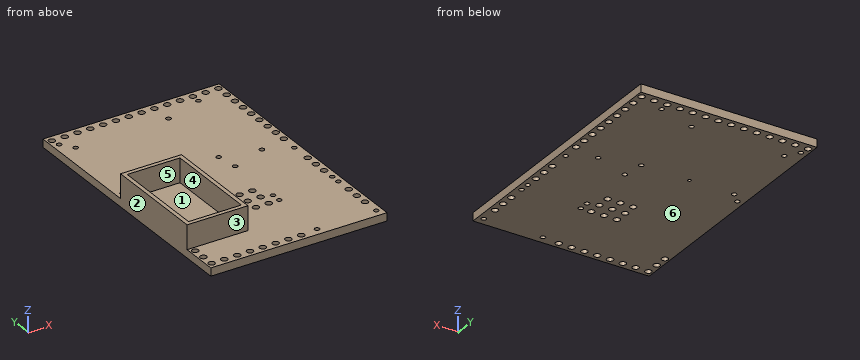
Autodesk Fusion 360 part; units mm, degrees
sketch "Skizze1" plane through (0, 0, 0) normal (0, 0, 1) x (1, 0, 0)
  line L0 (-55, 110) -> (55, 110)
  line L1 (55, 110) -> (55, -50)
  line L2 (55, -50) -> (-55, -50)
  line L3 (-55, -50) -> (-55, 110)
  circle A0 centre (0, 0) radius 2
  line L4 (0, 0) -> (-8, 0)
  line L5 (-8, 0) -> (-8, 8)
  line L6 (-8, 8) -> (0, 8)
  line L7 (0, 8) -> (0, 0)
  line L8 (-8, 8) -> (8, 8)
  line L9 (8, 8) -> (8, -8)
  line L10 (8, -8) -> (-8, -8)
  line L11 (-8, -8) -> (-8, 8)
  line L12 (0, 8) -> (8, 8)
  line L13 (8, 8) -> (8, -8)
  line L14 (8, -8) -> (0, -8)
  line L15 (0, -8) -> (0, 8)
  line L16 (-8, 0) -> (8, 0)
  line L17 (8, 0) -> (8, -8)
  line L18 (8, -8) -> (-8, -8)
  line L19 (-8, -8) -> (-8, 0)
  circle A1 centre (0, 8) radius 2
  circle A2 centre (-8, 8) radius 2
  circle A3 centre (-8, 0) radius 2
  circle A4 centre (-8, -8) radius 2
  circle A5 centre (0, -8) radius 2
  circle A6 centre (8, -8) radius 2
  circle A7 centre (8, 0) radius 2
  circle A8 centre (8, 8) radius 2
  circle A9 centre (-45.5, 97) radius 1.5
  circle A10 centre (12.5, 48) radius 1.5
  line L20 (-45.5, 97) -> (12.5, 97)
  line L21 (12.5, 97) -> (12.5, 48)
  line L22 (12.5, 48) -> (-45.5, 48)
  line L23 (-45.5, 48) -> (-45.5, 97)
  circle A11 centre (-45.5, 48) radius 1.5
  circle A12 centre (12.5, 97) radius 1.5
  line L24 (-50, 101.5) -> (35, 101.5)
  line L25 (35, 101.5) -> (35, 45.5)
  line L26 (35, 45.5) -> (-50, 45.5)
  line L27 (-50, 45.5) -> (-50, 101.5)
  line L28 (-45.5, 48) -> (12.5, 48)
  line L29 (12.5, 48) -> (12.5, 72.5)
  line L30 (-50, 45.5) -> (35, 45.5)
  line L31 (35, 45.5) -> (35, 73.5)
  line L32 (-51, 104.5) -> (36, 104.5)
  line L33 (36, 104.5) -> (36, 42.5)
  line L34 (36, 42.5) -> (-51, 42.5)
  line L35 (-51, 42.5) -> (-51, 104.5)
  circle A13 centre (-51, 42.5) radius 1.5
  circle A14 centre (-51, 104.5) radius 1.5
  circle A15 centre (36, 104.5) radius 1.5
  circle A16 centre (36, 42.5) radius 1.5
  line L36 (-7.5, 104.5) -> (-7.5, 42.5)
  line L37 (36, 73.5) -> (-51, 73.5)
  line L38 (-7.5, 101.5) -> (-7.5, 45.5)
  line L39 (35, 73.5) -> (-50, 73.5)
  line L40 (-52.5, 35.7098) -> (-19.5, 35.7098)
  line L41 (-19.5, 35.7098) -> (-19.5, -24.2902)
  line L42 (-19.5, -24.2902) -> (-52.5, -24.2902)
  line L43 (-52.5, -24.2902) -> (-52.5, 35.7098)
  line L44 (-36, 35.7098) -> (-36, -24.2902)
  line L45 (-19.5, 5.7098) -> (-52.5, 5.7098)
  line L46 (-55, 38.2098) -> (-17, 38.2098)
  line L47 (-17, 38.2098) -> (-17, -26.7902)
  line L48 (-17, -26.7902) -> (-55, -26.7902)
  line L49 (-55, -26.7902) -> (-55, 38.2098)
  line L50 (-36, 38.2098) -> (-36, -26.7902)
  line L51 (-17, 5.7098) -> (-55, 5.7098)
  line L52 (11.5, -5) -> (54.5, -5)
  line L53 (54.5, -5) -> (54.5, -48)
  line L54 (54.5, -48) -> (11.5, -48)
  line L55 (11.5, -48) -> (11.5, -5)
  line L56 (14.5, -8) -> (51.5, -8)
  line L57 (51.5, -8) -> (51.5, -45)
  line L58 (51.5, -45) -> (14.5, -45)
  line L59 (14.5, -45) -> (14.5, -8)
  circle A17 centre (14.5, -8) radius 1.5
  circle A18 centre (51.5, -8) radius 1.5
  circle A19 centre (51.5, -45) radius 1.5
  circle A20 centre (14.5, -45) radius 1.5
  line L60 (14.5, -26.5) -> (51.5, -26.5)
  line L61 (33, -8) -> (33, -45)
  line L62 (33, -5) -> (33, -48)
  line L63 (54.5, -26.5) -> (11.5, -26.5)
  line L64 (11.5, -5) -> (11.5, 38)
  circle A21 centre (14.5, -2) radius 1.5
  circle A22 centre (51.5, 35) radius 1.5
  circle A23 centre (14.5, 35) radius 1.5
  line L65 (11.5, 38) -> (54.5, 38)
  line L66 (33, 38) -> (33, -5)
  line L67 (54.5, 16.5) -> (11.5, 16.5)
  line L68 (33, 35) -> (33, -2)
  line L69 (14.5, 16.5) -> (51.5, 16.5)
  line L70 (14.5, 35) -> (51.5, 35)
  line L71 (54.5, -5) -> (11.5, -5)
  line L72 (51.5, 35) -> (51.5, -2)
  line L73 (54.5, 38) -> (54.5, -5)
  line L74 (51.5, -2) -> (14.5, -2)
  circle A24 centre (51.5, -2) radius 1.5
  line L75 (14.5, -2) -> (14.5, 35)
  line L76 (33, 16.5) -> (33, -26.5)
  line L77 (-55, 110) -> (55, 110)
  line L78 (55, 110) -> (55, 104.5)
  line L79 (55, 104.5) -> (-55, 104.5)
  line L80 (-55, 104.5) -> (-55, 110)
  line L81 (-55, 104.5) -> (-7.5, 104.5)
  line L82 (-7.5, 104.5) -> (-7.5, 73.5)
  line L83 (-7.5, 73.5) -> (-55, 73.5)
  line L84 (-55, 73.5) -> (-55, 104.5)
  line L85 (-55, 42.7098) -> (-36, 42.7098)
  line L86 (-36, 42.7098) -> (-36, 5.7098)
  line L87 (-36, 5.7098) -> (-55, 5.7098)
  line L88 (-55, 5.7098) -> (-55, 42.7098)
  line L89 (55, 42.5) -> (33, 42.5)
  line L90 (33, 42.5) -> (33, 16.5)
  line L91 (33, 16.5) -> (55, 16.5)
  line L92 (55, 16.5) -> (55, 42.5)
  line L93 (-55, 110) -> (55, 110)
  line L94 (55, 110) -> (55, 114)
  line L95 (55, 114) -> (-55, 114)
  line L96 (-55, 114) -> (-55, 110)
  circle A25 centre (-28, 110) radius 2
  circle A26 centre (-20, 110) radius 2
  circle A27 centre (-12, 110) radius 2
  circle A28 centre (-36, 110) radius 2
  circle A29 centre (-44, 110) radius 2
  circle A30 centre (-52, 110) radius 2
  circle A31 centre (-4, 110) radius 2
  circle A32 centre (4, 110) radius 2
  circle A33 centre (12, 110) radius 2
  circle A34 centre (20, 110) radius 2
  circle A35 centre (28, 110) radius 2
  circle A36 centre (36, 110) radius 2
  circle A37 centre (44, 110) radius 2
  circle A38 centre (52, 110) radius 2
  line L97 (52, 110) -> (52, 42.5)
  circle A39 centre (52, 102) radius 2
  circle A40 centre (52, 94) radius 2
  circle A41 centre (52, 86) radius 2
  circle A42 centre (52, 70) radius 2
  circle A43 centre (52, 78) radius 2
  circle A44 centre (52, 62) radius 2
  circle A45 centre (52, 54) radius 2
  circle A46 centre (52, 46) radius 2
  line L98 (-55, -50) -> (11.5, -50)
  line L99 (11.5, -50) -> (11.5, -46)
  line L100 (11.5, -46) -> (-55, -46)
  line L101 (-55, -46) -> (-55, -50)
  circle A47 centre (-52, -46) radius 2
  circle A48 centre (-44, -46) radius 2
  circle A49 centre (-36, -46) radius 2
  circle A50 centre (-28, -46) radius 2
  circle A51 centre (-20, -46) radius 2
  circle A52 centre (-12, -46) radius 2
  circle A53 centre (-4, -46) radius 2
  circle A54 centre (4, -46) radius 2
  circle A55 centre (-17.5, 48) radius 1
  line L102 (-52, -46) -> (-52, -24.2902)
  circle A56 centre (-52, -38) radius 2
  circle A57 centre (-52, -30) radius 2
  circle A58 centre (51.5, 22) radius 2
  circle A59 centre (51.5, 14) radius 2
  circle A60 centre (51.5, 6) radius 2
  circle A61 centre (51.5, -18) radius 2
  circle A62 centre (51.5, -26) radius 2
  circle A63 centre (51.5, -34) radius 2
  point P0 (-7.5, 73.5)
  point P1 (-7.5, 73.5)
  point P2 (-36, 5.7098)
  point P3 (-36, 5.7098)
  point P4 (33, -26.5)
  point P5 (33, -26.5)
  point P6 (33, 16.5)
  point P7 (33, 16.5)
  point P8 (-52, 110)
  point P9 (-44, 110)
  point P10 (-36, 110)
  dimension "d1" = 110
  dimension "d2" = 160
  dimension "d3" = 55
  dimension "d4" = 50
  dimension "d5" = 4
  dimension "d6" = 8
  dimension "d7" = 8
  dimension "d8" = 16
  dimension "d9" = 16
  dimension "d10" = 4
  dimension "d11" = 4
  dimension "d12" = 4
  dimension "d13" = 4
  dimension "d14" = 4
  dimension "d15" = 4
  dimension "d16" = 4
  dimension "d17" = 4
  dimension "d20" = 3
  dimension "d23" = 3
  dimension "d28" = 3
  dimension "d29" = 3
  dimension "d30" = 58
  dimension "d31" = 49
  dimension "d32" = 85
  dimension "d33" = 56
  dimension "d35" = 4.5
  dimension "d36" = 4.5
  dimension "d37" = 87
  dimension "d38" = 62
  dimension "d39" = 3
  dimension "d40" = 3
  dimension "d41" = 3
  dimension "d42" = 3
  dimension "d45" = 33
  dimension "d46" = 60
  dimension "d47" = 38
  dimension "d48" = 65
  dimension "d51" = 43
  dimension "d52" = 43
  dimension "d53" = 37
  dimension "d54" = 37
  dimension "d55" = 3
  dimension "d56" = 3
  dimension "d57" = 3
  dimension "d58" = 3
  dimension "d59" = 43
  dimension "d60" = 43
  dimension "d61" = 37
  dimension "d62" = 37
  dimension "d63" = 3
  dimension "d64" = 3
  dimension "d65" = 3
  dimension "d66" = 3
  dimension "d67" = 43
  dimension "d68" = 5.5
  dimension "d69" = 47.5
  dimension "d70" = 31
  dimension "d71" = 19
  dimension "d72" = 37
  dimension "d73" = 22
  dimension "d74" = 26
  dimension "d75" = 4
  dimension "d76" = 3
  dimension "d77" = 8
  dimension "d78" = 8
  dimension "d79" = 4
  dimension "d80" = 4
  dimension "d81" = 4
  dimension "d82" = 8
  dimension "d83" = 8
  dimension "d84" = 8
  dimension "d85" = 4
  dimension "d86" = 4
  dimension "d87" = 4
  dimension "d88" = 4
  dimension "d89" = 4
  dimension "d90" = 4
  dimension "d91" = 4
  dimension "d92" = 8
  dimension "d93" = 8
  dimension "d94" = 8
  dimension "d95" = 8
  dimension "d96" = 4
  dimension "d97" = 4
  dimension "d98" = 4
  dimension "d99" = 4
  dimension "d100" = 8
  dimension "d101" = 8
  dimension "d102" = 8
  dimension "d103" = 8
  dimension "d104" = 4
  dimension "d105" = 4
  dimension "d106" = 4
  dimension "d107" = 4
  dimension "d108" = 4
  dimension "d110" = 4
  dimension "d111" = 4
  dimension "d112" = 8
  dimension "d113" = 8
  dimension "d114" = 8
  dimension "d116" = 8
  dimension "d117" = 8
  dimension "d118" = 8
  dimension "d119" = 8
  dimension "d120" = 4
  dimension "d121" = 8
  dimension "d122" = 4
  dimension "d123" = 4
  dimension "d124" = 4
  dimension "d125" = 4
  dimension "d126" = 4
  dimension "d127" = 3
  dimension "d128" = 8
  dimension "d129" = 8
  dimension "d130" = 8
  dimension "d131" = 4
  dimension "d132" = 4
  dimension "d133" = 4
  dimension "d134" = 8
  dimension "d135" = 8
  dimension "d136" = 8
  dimension "d137" = 4
  dimension "d138" = 8
  dimension "d139" = 2
  dimension "d140" = 28
  dimension "d141" = 4
  dimension "d142" = 4
  dimension "d143" = 8
  dimension "d144" = 8
  dimension "d145" = 4
  dimension "d146" = 24
  dimension "d147" = 4
  dimension "d148" = 8
  dimension "d149" = 4
  dimension "d150" = 8
  dimension "d151" = 4
  dimension "d152" = 4
  dimension "d153" = 4
  dimension "d154" = 24
  dimension "d155" = 8
  dimension "d156" = 8
extrude "Extrusion2" add sketch "Skizze1" along normal blind 5 contours L0 L77 L93 L94 L95 L96 A25 A26 A27 A28 A29 A30 A31 A32 A33 A34 A35 A36 A37 A38 | L0 L1 L77 L78 L79 L93 A38 L97 | L0 L3 L32 A14 A15 L77 L79 L80 L81 L93 A25 A26 A27 A28 A29 A30 A31 A32 A33 A34 A35 A36 A37 A38 L97 | L33 A15 A16 L79 L89 L97 A39 A40 A41 A42 A43 A44 A45 A46 | L1 L79 L89 L97 A39 A40 A41 A42 A43 A44 A45 A46 | L1 L34 A16 L65 L73 L89 L90 L91 L92 | L24 L25 L32 L33 A15 L36 L37 L79 L82 | L1 L2 L53 L54 L73 L91 L99 | L24 L27 L32 L35 A14 L36 L37 L79 L81 L82 L83 | L25 L26 L30 L31 L33 L34 A16 L36 L37 L89 | L52 L66 L67 L71 L72 L73 L74 A24 L76 L91 A59 A60 | A22 L65 L66 L67 L70 L72 L73 L90 L91 A58 | L3 L35 A14 L79 L81 L83 L84 | A9 L20 L23 L24 L27 L36 L37 L38 L39 L82 L83 | L20 L21 A12 L24 L25 L36 L37 L38 L39 L82 | A10 L21 L22 L25 L26 L28 L29 L30 L31 L36 L37 L38 L39 | L2 L3 L55 L98 L99 L100 L101 A47 A48 A49 A50 A51 A52 A53 A54 | L66 L67 L68 L69 L72 L74 A24 L76 L91 A59 A60 | A22 L66 L67 L68 L69 L70 L72 L90 L91 A58 | L52 L53 L56 L57 A18 L62 L63 L71 L76 A61 A62 | L3 L35 A13 L83 L85 | A9 L20 L23 L36 L37 L38 L39 L82 L83 | L20 L21 A12 L36 L37 L38 L39 L82 | A10 L21 L22 L28 L29 L36 L37 L38 L39 | L54 L55 L58 L59 A20 L62 L63 L99 | A23 L66 L67 L68 L69 L70 L75 L90 | A21 L66 L67 L68 L69 L74 L75 L76 | L64 A23 L65 L66 L67 L70 L75 L90 | L34 L46 L47 L48 L55 L64 L65 L86 L90 L100 A47 A48 A49 A50 A51 A52 A53 A54 L102 A56 A57 | L52 L55 L56 L59 A17 L62 L63 L71 L76 | L52 L64 A21 L66 L67 L71 L74 L75 L76 | L53 L54 L57 L58 A19 L62 L63 A62 A63 | L3 L34 A13 L46 L85 L86 L88 | L26 L27 L30 L34 L35 A13 L36 L37 L83 L85 L86 | L22 L23 A11 L26 L27 L28 L30 L36 L37 L38 L39 L83 A55 | L22 L23 A11 L28 L36 L37 L38 L39 L83 A55 | L3 L48 L100 A47 L102 A56 A57 | L56 L59 A17 L60 L61 L62 L63 L76 | L56 L57 A18 L60 L61 L62 L63 L76 A61 A62 | L3 L40 L43 L46 L49 L50 L51 L86 L87 L88 | L3 L42 L43 L48 L49 L51 L87 L102 | L57 L58 A19 L60 L61 L62 L63 A62 A63 | L58 L59 A20 L60 L61 L62 L63 | L34 A13 L85 L86 | L40 L41 L46 L47 L50 L51 L86 | L42 L48 L50 L102 | L42 L43 L44 L45 L50 L51 L87 | L40 L43 L44 L45 L50 L51 L86 L87 | L40 L41 L44 L45 L50 L51 L86 | L41 L42 L47 L48 L50 L51 | L41 L42 L44 L45 L50 L51 | A0 L9 L10 L13 L14 L15 L16 L17 L18 A5 A6 A7 | A0 L7 L8 L9 L12 L13 L15 L16 A1 A7 A8 | A0 L4 L5 L6 L7 L8 L11 L15 L16 A1 A2 A3 | A0 L4 L10 L11 L15 L16 L18 L19 A3 A4 A5
extrude "Extrusion3" add sketch "Skizze1" along normal blind 20 contours L3 L40 L43 L46 L49 L50 L51 L86 L87 L88 | L3 L42 L43 L48 L49 L51 L87 L102 | L40 L41 L46 L47 L50 L51 L86 | L42 L48 L50 L102 | L41 L42 L47 L48 L50 L51
Here's how the part is built. I have some questions about the finished solid (model axes, mm). Face numbers are marked on the shaded views. A direction names the side the tool comes from. Give positions to 0.01 mm unless a question says otherwise; leave off trailing zeros. Loops run counter-clockwise (first coordinate to the right, second up) from the corner with the lowest first, then second, coordinate; pieces in that order, holes last. Notation, with made-up numbers: M 26,70 L 85,70 A25 ccw 85,84 Z; hole C 69,27 d6. An arc over 180 degrees is marked long. Return JSON: item names as keys, results as strings.
Item 1: I'm going to push flat-ended pins straight in: pin 1 Ø1 at (x, y) = (-7.5, 82) entering from +Z; pin 2 Ø5 at (x, y) = (-52, 110) entering from -Z. Where does each tip first touch, or does it pass through?
A:
{"pin 1": "stops at z = 5", "pin 2": "stops at z = 0"}
Item 2: On a 3-axis mill with a long thin cutter (end or side, diameter ignored), from which of +Z, -Z, +X, -X, +Y, -Y can I reach the whole of each face in a straight line? I mean the marked faces 5 and 6. Say none if no direction works.
A:
{"face 5": "+Z", "face 6": "-Z, +X, -X, +Y, -Y"}
Item 3: Thinking about a two-plate mould opening in X: for the marked faces 1, 2, 3 and 4, which applies, released by +X, released by -X, zero draft, split by the parting line, or undercut?
A:
{"face 1": "undercut", "face 2": "released by -X", "face 3": "zero draft", "face 4": "undercut"}
Item 4: Please list where these lines run through material, in increasing order: line 1 (Y direction, x = -12, z = 2.5); line 2 (X direction, y = -8, z = 2.4); line 3 (X direction, y = -2.5, z = 8.75).
A:
{"line 1": "y = -50 to -48, -44 to 108, 112 to 114", "line 2": "x = -55 to -10, -6 to -2, 2 to 6, 10 to 13, 16 to 50, 53 to 55", "line 3": "x = -55 to -52.5, -19.5 to -17"}
Item 5: Imagine slicing it at A-A on y = 62. List the corners of the cut face in (x, z) for me.
A:
{"outline": "M -55,0 L 50,0 L 50,5 L -55,5 Z; M 54,0 L 55,0 L 55,5 L 54,5 Z"}
Item 6: Imagine slicing it at B-B on x = -4. List the corners of the cut face in (y, z) for me.
A:
{"outline": "M -50,0 L -48,0 L -48,5 L -50,5 Z; M -44,0 L 108,0 L 108,5 L -44,5 Z; M 112,0 L 114,0 L 114,5 L 112,5 Z"}
Item 7: Imagine slicing it at C-C on z = 11.25. List the corners of the cut face in (x, y) for me.
A:
{"outline": "M -55,-26.79 L -17,-26.79 L -17,38.21 L -55,38.21 Z; hole M -52.5,-24.29 L -19.5,-24.29 L -19.5,35.71 L -52.5,35.71 Z"}
